Geometry: final body of the model. Coordinates: model frame, mm. Face numbers are marked on the shaded views. A direction names the side the tool comes from. Give positions to 0.01 mm unless a question says otherwise; leave off trailing zeros. Loops run counter-clockwise (first coordinate to the right, second up) from the corner with the lowest first, then second, coordinate; pieces in that order, holes last. Notation, with made-up numbers: (-3, 4.25) -> (45, 4.25) arc R20 cw to (45, 24.25) -> close; hole circle Ø7 at (-34.5, 31.5). An arc over 180 degrees is marked (long way). Answer in a Markdown table with one row per item. Add a question column.
1) First-contact query: P1, Ø9.5, axis at y = 7.5, z = 30.5, coming from the +X side; P2, Ø5.5, axis at x = 68.5, y = 13, coming from the +Z side; P3, Ø4, axis at x = 92.5, y = 5, coming from the -Z side. Flat tips, straight axial feed; report the tip coordinate or a pass-through.
2) Section query B-B (y = 13.75). Return the cut outline in (x, z), plus the area to 3 significant figures.
3) Section query A-A (z = 4.47). Return the cut outline in (x, y), plus the area to 3 significant figures.
4) Line query: line 1 (Z direction, x = 66.5, y = 7.75); line 2 (X direction, y = 6.5, z = 48.26); line 3 (Z direction, x = 4, y = 9). Output: solid intervals per line, ascending. Write a range as from..to.
5) Section query C-C (x = 50.5). Return the cut outline in (y, z), plus the area to 3 significant figures.
6) Access query for the marked faces 1, 2, 3, 4 and 5. Directions: +Z, -Z, +X, -X, +Y, -Y. A direction counts if a zero-diameter tool reaches every point of the face in a straight line with its end or side. Return the directions, or none.
7) Section query D-D (z = 39). Return the cut outline in (x, y), plus the area to 3 significant figures.
```python
from build123d import *

# Parameters (mm, degrees)
SKETCH1_R           = 1.5
BOSS_EXTRUDE1_DEPTH = 18.86
SKETCH2_W           = 100
SKETCH2_H           = 90
BOSS_EXTRUDE2_DEPTH = 1


with BuildPart() as part:
    # Sketch1 → Boss-Extrude1 (new body)
    with BuildSketch(Plane(origin=(0, 0, 0), x_dir=(1, 0, 0), z_dir=(0, 1, 0))):
        Polygon((0, 0), (0, -57.76), (108.8, -57.76), (113.8, -54.88), (113.8, -14.88), (108.8, -12), (108.8, 0), align=None)
        with Locations(Location((66.5, -9.5, 0), (0, 0, 90))):
            Circle(SKETCH1_R, mode=Mode.SUBTRACT)
        with Locations(Location((4, -4.47, 0), (0, 0, 90))):
            Circle(SKETCH1_R, mode=Mode.SUBTRACT)
        with Locations(Location((3.8, -53.57, 0), (0, 0, 90))):
            Circle(SKETCH1_R, mode=Mode.SUBTRACT)
        with Locations(Location((66.5, -48.26, 0), (0, 0, 90))):
            Circle(SKETCH1_R, mode=Mode.SUBTRACT)
    extrude(amount=BOSS_EXTRUDE1_DEPTH)

    # Sketch2 → Boss-Extrude2 (add)
    with BuildSketch(Plane(origin=(0, 18.86, 0), x_dir=(1, 0, 0), z_dir=(0, 1, 0))):
        with Locations((73.8, -25.76)):
            Rectangle(SKETCH2_W, SKETCH2_H)
    extrude(amount=BOSS_EXTRUDE2_DEPTH)


solid = part.part
```
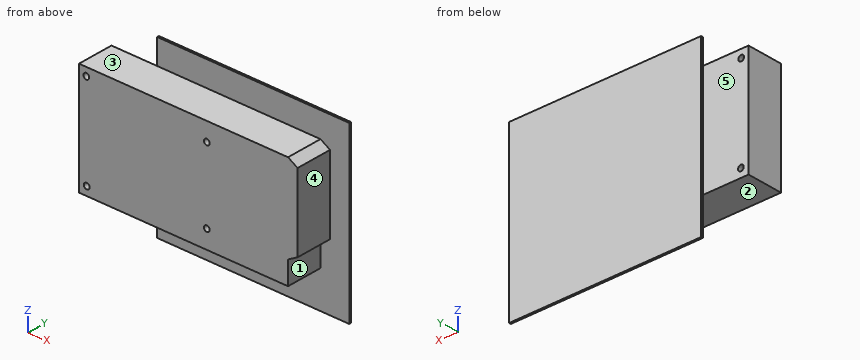
Evaluation:
| question | item | result |
|---|---|---|
| 1 | P1 | x = 113.8 |
| 1 | P2 | z = 57.76 |
| 1 | P3 | z = 0 |
| 2 | outline | (0, 0) -> (108.8, 0) -> (108.8, 12) -> (113.8, 14.88) -> (113.8, 54.88) -> (108.8, 57.76) -> (0, 57.76) -> close; hole circle Ø3 at (3.8, 53.57); hole circle Ø3 at (4, 4.47); hole circle Ø3 at (66.5, 9.5); hole circle Ø3 at (66.5, 48.26) |
| 2 | area | 6,470 mm² |
| 3 | outline | (0, 0) -> (2.5, 0) -> (2.5, 18.86) -> (0, 18.86) -> close; (5.5, 0) -> (108.8, 0) -> (108.8, 18.86) -> (123.8, 18.86) -> (123.8, 19.86) -> (23.8, 19.86) -> (23.8, 18.86) -> (5.5, 18.86) -> close |
| 3 | area | 2,100 mm² |
| 4 | line 1 | 0..8, 11..46.76, 49.76..57.76 |
| 4 | line 2 | 0..65, 68..113.8 |
| 4 | line 3 | 0..2.97, 5.97..52.08, 55.06..57.76 |
| 5 | outline | (0, 0) -> (18.86, 0) -> (18.86, -19.24) -> (19.86, -19.24) -> (19.86, 70.76) -> (18.86, 70.76) -> (18.86, 57.76) -> (0, 57.76) -> close |
| 5 | area | 1,180 mm² |
| 6 | face 1 | -Z, +X, -Y |
| 6 | face 2 | -Z, +X, -X, -Y |
| 6 | face 3 | +Z, +X, -X, -Y |
| 6 | face 4 | +Z, -Z, +X, -Y |
| 6 | face 5 | +Z, -Z, -X, +Y |
| 7 | outline | (0, 0) -> (113.8, 0) -> (113.8, 18.86) -> (123.8, 18.86) -> (123.8, 19.86) -> (23.8, 19.86) -> (23.8, 18.86) -> (0, 18.86) -> close |
| 7 | area | 2,250 mm² |
